Part model, mm, in its own coordinate system. A direction names the side the tool comes from. Round coordinates to 2 decimals unless told otherwise and drop trailing zeros. Write each loop counter-clockwise with the first axis right and the second up, starting at its lowest first coordinate (ties: lowest second). Pieces come first, ordered by that corner, then holes. Notation, with made-up numbers: M 48.5,-12.75 L 106.5,-12.75 A8 cw 106.5,-5.75 Z; hole C -10,31 d1. An arc over 180 degrees is marked long. Use one line per item in the form item = value. Start each with the question number.
Item 1: Mould opens along X. For faces 4 (the face through (0, 2, -11)), 5 (the face through (12, 2, -11)), 6 (the face through (6, 0, -11)), 7 (the face through (6, 2, 0)) say: +X half, -X half, draft (parallel to the pull), parting line (faces both ways), or undercut.
Item 2: Probe L1, parallel to X at y = 4.3, z = -16; L2, parallel to X at y = 2.3, z = -16; L3, parallel to Y at x = 2.5, z = -17.75. List the from-to ranges inside material, lowest first.
Item 3: Flat gauge pins, fed straight in: pin 1 Ø5 at (x, z) = (6, -16) entering from +Y; pin 2 Ø3 at (x, z) = (6, -5) entering from -Y; pin 3 Ø4 at (x, z) = (6, -17.5) entering from +Y; pin 4 Ø1.5 at (x, y) = (7, 2.5) entering from +Z. Where does each tip first touch, or does it go through?
Item 4: Cut at A-A, the plane y = 2.5. Give the cut face in (x, z), then the cut area to 3 significant figures.
Item 5: Which spindle directions (+Z, -Z, +X, -X, +Y, -Y) get a long thin tool onto all of the face, cutting with end or side? Do faces 1 (the face through (2, 2, 2)), 2 (the face through (11.11, 1.49, 0.99)), 3 (the face through (3, 3, -15)). Say none if no direction does.
Item 6: Cut at D-D, the plane z = -12.75. Give the cut face in (x, y), then the cut area to 3 significant figures.
Item 7: Cut at B-B, the plane x = 8. Give the cut face in (y, z).
Item 8: Cut at C-C, the plane z = -17.25. Give the cut face in (x, y), then the cut area to 3 significant figures.
from build123d import *

# Parameters (mm, degrees)
SKETCH_1_W      = 12
SKETCH_1_H      = 22
SKETCH_1_R      = 2.9
EXTRUDE_1_DEPTH = 3
SKETCH_3_W      = 12
SKETCH_3_H      = 22
SKETCH_3_R      = 4.1
EXTRUDE_2_DEPTH = 2
SKETCH_7_R      = 1.5
EXTRUDE_3_DEPTH = 2


with BuildPart() as part:
    # 草图1 → 凸台-拉伸1 (new body)
    with BuildSketch(Plane(origin=(0, 0, 0), x_dir=(1, 0, 0), z_dir=(0, 1, 0))):
        with Locations((6, 11)):
            Rectangle(SKETCH_1_W, SKETCH_1_H)
        with Locations(Location((6, 16, 0), (0, 0, 270))):
            Circle(SKETCH_1_R, mode=Mode.SUBTRACT)
    extrude(amount=EXTRUDE_1_DEPTH)

    # 草图3 → 凸台-拉伸2 (add)
    with BuildSketch(Plane(origin=(0, 3, 0), x_dir=(1, 0, 0), z_dir=(0, 1, 0))):
        with Locations((6, 11)):
            Rectangle(SKETCH_3_W, SKETCH_3_H)
        with Locations(Location((6, 16, 0), (0, 0, 270))):
            Circle(SKETCH_3_R, mode=Mode.SUBTRACT)
    extrude(amount=EXTRUDE_2_DEPTH)

    # 草图7 → 凸台-拉伸3 (add)
    with BuildSketch(Plane.XY):
        with Locations(Location((2, 2.5, 0), (0, 0, 180))):
            Circle(SKETCH_7_R)
        with Locations(Location((10, 2.5, 0), (0, 0, 180))):
            Circle(SKETCH_7_R)
    extrude(amount=EXTRUDE_3_DEPTH)


solid = part.part
Model answer:
q1.face_4 = -X half
q1.face_5 = +X half
q1.face_6 = draft
q1.face_7 = undercut
q2.L1 = 0 to 1.9, 10.1 to 12
q2.L2 = 0 to 3.1, 8.9 to 12
q2.L3 = 0 to 3
q3.pin_1 = through
q3.pin_2 = 0
q3.pin_3 = 3
q3.pin_4 = 0
q4.outline = M 0,-22 L 12,-22 L 12,0 L 11.5,0 L 11.5,2 L 8.5,2 L 8.5,0 L 3.5,0 L 3.5,2 L 0.5,2 L 0.5,0 L 0,0 Z; hole C 6,-16 d5.8
q4.area = 250 mm²
q5.face_1 = +Z, +X, -X, +Y, -Y
q5.face_2 = +Z
q5.face_3 = +Y
q6.outline = M 0,0 L 12,0 L 12,5 L 8.5,5 L 8.5,3 L 3.5,3 L 3.5,5 L 0,5 Z
q6.area = 50.0 mm²
q7.outline = M 0,-22 L 5,-22 L 5,-19.58 L 3,-19.58 L 3,-18.1 L 0,-18.1 Z; M 0,-13.9 L 3,-13.9 L 3,-12.42 L 5,-12.42 L 5,0 L 0,0 Z
q8.outline = M 0,0 L 3.38,0 L 3.38,3 L 2.1,3 L 2.1,5 L 0,5 Z; M 8.62,0 L 12,0 L 12,5 L 9.9,5 L 9.9,3 L 8.62,3 Z
q8.area = 28.7 mm²
